Can you work these out from the model? Positions are in its coordinate system, mm. Coordinates: 2 decimals unless noted, no trailing zeros. Order: outer loops, then holes, each group sorted by start corner. A loop starts at its lowest first (then second) coordinate and runs counter-clockwise, first axis right, second up. Notation, with made-up numbers: (-36, 18.25) -> (8, 18.25) arc R23 ccw to (8, 39.25) -> close; hole circle Ø10 at (13, 78). An arc over 180 degrees is marked (long way). Answer as CSV lines item,"result".
from build123d import *

# Parameters (mm, degrees)
SKETCH_1_W      = 151.6
SKETCH_1_H      = 186.8
SKETCH_1_W_2    = 30.4
SKETCH_1_H_2    = 4.4
SKETCH_1_W_3    = 4
SKETCH_1_H_3    = 30
SKETCH_1_W_4    = 30
SKETCH_1_H_4    = 4
EXTRUDE_1_DEPTH = 3


with BuildPart() as part:
    # Эскиз1 → Бобышка-Вытянуть1 (new body)
    # profile 1 of 7: a face of its own
    with BuildSketch(Plane.XY):
        with Locations((75.8, 93.4)):
            Rectangle(SKETCH_1_W, SKETCH_1_H)
        with Locations((25.8, 8)):
            Rectangle(SKETCH_1_W_2, SKETCH_1_H_2, mode=Mode.SUBTRACT)
        with Locations((125.8, 8)):
            Rectangle(SKETCH_1_W_2, SKETCH_1_H_2, mode=Mode.SUBTRACT)
    # profile 2 of 7: a face of its own
    with BuildSketch(Plane.XY):
        with Locations((-2, 43.4)):
            Rectangle(SKETCH_1_W_3, SKETCH_1_H_3)
    # profile 3 of 7: a face of its own
    with BuildSketch(Plane.XY):
        with Locations((-2, 143.4)):
            Rectangle(SKETCH_1_W_3, SKETCH_1_H_3)
    # profile 4 of 7: a face of its own
    with BuildSketch(Plane.XY):
        with Locations((153.6, 143.4)):
            Rectangle(SKETCH_1_W_3, SKETCH_1_H_3)
    # profile 5 of 7: a face of its own
    with BuildSketch(Plane.XY):
        with Locations((153.6, 43.4)):
            Rectangle(SKETCH_1_W_3, SKETCH_1_H_3)
    # profile 6 of 7: a face of its own
    with BuildSketch(Plane.XY):
        with Locations((35.8, 188.8)):
            Rectangle(SKETCH_1_W_4, SKETCH_1_H_4)
    # profile 7 of 7: a face of its own
    with BuildSketch(Plane.XY):
        with Locations((115.8, 188.8)):
            Rectangle(SKETCH_1_W_4, SKETCH_1_H_4)
    extrude(amount=EXTRUDE_1_DEPTH)


solid = part.part
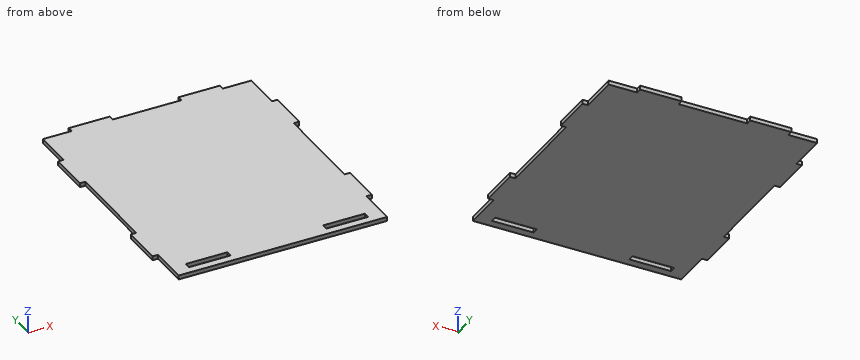
Q1. Imagine slicing it at A-A (x = 113). List the corners of the cut face in (y, z) for me, and give its area (3 significant figures).
Solution:
outline,"(0, 0) -> (5.8, 0) -> (5.8, 3) -> (0, 3) -> close; (10.2, 0) -> (190.8, 0) -> (190.8, 3) -> (10.2, 3) -> close"
area,"559 mm2"
Q2. Imagine slicing it at C-C (y = 81). List the corners of the cut face in (x, z) for me, and give its area (3 significant figures).
Solution:
outline,"(0, 0) -> (151.6, 0) -> (151.6, 3) -> (0, 3) -> close"
area,"455 mm2"
Q3. If I drill on line 1 (X direction, y = 8, z = 1.4); line 2 (Y direction, x = 134.5, z = 1.4); line 3 (Y direction, x = 128, z = 0.8), over which ranges is the centre line in solid material (lowest first)?
Solution:
line 1,"0 to 10.6, 41 to 110.6, 141 to 151.6"
line 2,"0 to 5.8, 10.2 to 186.8"
line 3,"0 to 5.8, 10.2 to 190.8"
Q4. Imagine slicing it at D-D (x = 85). List the corners of the cut face in (y, z) for me.
Solution:
outline,"(0, 0) -> (186.8, 0) -> (186.8, 3) -> (0, 3) -> close"
Q5. For P1, Ø1.5, axis at x = 137, z = 2, coming from the +Y side; P2, Ø1.5, axis at y = 16.5, z = 1.5, coming from the +X side; P3, Ø1.5, axis at x = -3, z = 1.5, coming from the -Y side, each with a flat end and sliding along its axis, tell me the tip position at first contact or that it passes through.
Solution:
P1,"y = 186.8"
P2,"x = 151.6"
P3,"y = 28.4"
Q6. Imagine slicing it at B-B (z = 1.4). Give the number of separate pieces and of enclosed holes in the cut face, and give its area (3 significant figures).
Solution:
separate pieces,"1"
enclosed holes,"2"
area,"28,800 mm2"
